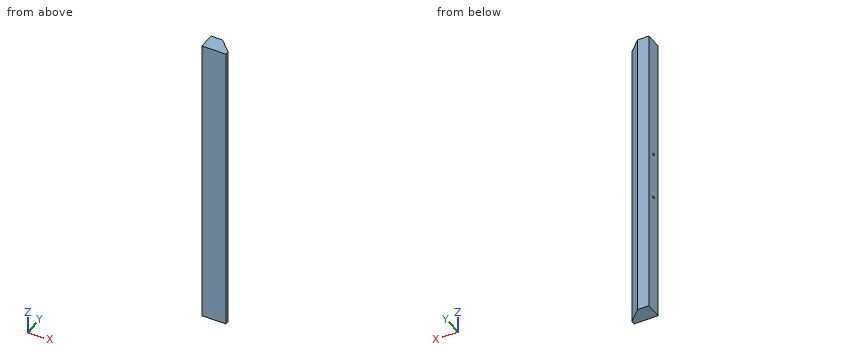
from build123d import *

# Parameters (mm, degrees)
BOSS_EXTRUDE1_DEPTH = 1828.8
SKETCH3_R           = 8.5725
CUT_EXTRUDE2_DEPTH  = 63.5


with BuildPart() as part:
    # Sketch1 → Boss-Extrude1 (new body)
    with BuildSketch(Plane.XY):
        Polygon((4.233333333, 36.865277778), (83.608333333, -40.745833333), (83.608333333, -64.734722222), (-65.616666667, -64.734722222), (-65.616666667, 36.865277778), align=None)
    extrude(amount=BOSS_EXTRUDE1_DEPTH)

    # Sketch3 → Cut-Extrude2 (cut)
    with BuildSketch(Plane.ZY.offset(65.616666667)):
        with Locations((769.62, -13.934722222)):
            Circle(SKETCH3_R)
        with Locations(Location((1059.18, -13.934722222, 0), (0, 0, 180))):
            Circle(SKETCH3_R)
    extrude(amount=-CUT_EXTRUDE2_DEPTH, mode=Mode.SUBTRACT)


solid = part.part
The model under review builds one solid part; all positions refer to its coordinate system, in mm. Round coordinates to 2 decimals unless told otherwise and drop trailing zeros. Order: outer loops, then holes, each group sorted by start corner. A loop starts at its lowest first (then second) coordinate and runs counter-clockwise, first axis right, second up. Notation, with made-up numbers: (-35.5, 86) - (22.5, 86) arc R18 cw to (22.5, 106) - close; hole circle Ø9 at (42, 51.5). An arc over 180 degrees is marked (long way). Use one line per item in the form item = value.
Q1. Clearance check with flat-ended pins moving along their axes: P1, Ø13.5, axis at y = -13.93, z = 1059.18, coming from the +X side; P2, Ø12, axis at x = 31, z = 1146, coming from the +Y side. State where each tip first meets the part, or that it passes through.
Response values:
P1 = 63.09
P2 = 16.56
Q2. Add section C-C on y = 18. Give the boundary of the cut face in (x, z), then the cut area to 3 significant figures.
Response values:
outline = (-65.62, 0) - (23.53, 0) - (23.53, 1828.8) - (-65.62, 1828.8) - close
area = 163,000 mm^2
Q3. Add section B-B on x = 50. Give the boundary of the cut face in (y, z), then the cut area to 3 significant figures.
Response values:
outline = (-64.73, 0) - (-7.88, 0) - (-7.88, 1828.8) - (-64.73, 1828.8) - close
area = 104,000 mm^2
Q4. To check wall thickness, follow line 1 (Y direction, x = -50.5, z = 769.62); line 2 (Z direction, x = -30, y = -6.5); line 3 (X direction, y = -13, z = 1639). State the ranges of each line that lie inside material, in increasing order.
Response values:
line_1 = -64.73 to -22.51, -5.36 to 36.87
line_2 = 0 to 765.35, 773.89 to 1054.91, 1063.45 to 1828.8
line_3 = -65.62 to 55.23
Q5. Add section A-A on z = 969. Give the boundary of the cut face in (x, y).
Response values:
outline = (-65.62, -64.73) - (83.61, -64.73) - (83.61, -40.75) - (4.23, 36.87) - (-65.62, 36.87) - close
